Read the model definition and answer for the solid it produces. Units are mm, in the model's axes. Coordinates: 2 decimals unless noted, no trailing zeros. Write each loop counter-clockwise with the first axis right and the second up, starting at its lowest first coordinate (ties: lowest second). Pieces come first, ordered by that corner, then holes.
(1) Given pin 1 (1 mm diameter, centred on x = -2.5, y = 0.5, fed in from +Z); pin 2 (1 mm diameter, centred on x = -8, y = 2.5, fed in from -Z), each flat-ended and moving along its own axis, determine where each tip first touches the part or whether it passes through.
(2) Find the intervals of material crossed by probe 1 along Z at (x, y) = (-21.5, 1.8); probe 2 along Z at (x, y) = (-3, 1.55); probe 3 along X at (y, z) = (0.6, -132.5), in increasing order.
(3) Section B-B on x = -26.5 is taken. Write down the section's boundary in (y, z).
Autodesk Inventor part; units mm, degrees
ref_plane "YZ Plane" through (0, 0, 0) normal (1, 0, 0) x (0, 1, 0)
ref_plane "XZ Plane" through (0, 0, 0) normal (0, 1, 0) x (-1, 0, 0)
ref_plane "XY Plane" through (0, 0, 0) normal (0, 0, 1) x (1, 0, 0)
sketch "Sketch1" plane through (0, 0, 0) normal (0, 1, 0) x (-1, 0, 0)
  line L0 (0, 0) -> (-30, 0)
  line L1 (-30, 0) -> (-30, -140)
  line L2 (-30, -140) -> (0, -140)
  line L3 (0, -140) -> (0, 0)
  line L4 (0, 0) -> (0, -10)
  line L5 (0, -10) -> (40, -10)
  line L6 (40, -10) -> (40, -130)
  line L7 (40, -130) -> (0, -130)
  line L8 (0, -130) -> (0, -10)
  point P0 (0, -130)
  dimension "d0" = 30
  dimension "d1" = 140
  dimension "d2" = 10
  dimension "d3" = 40
  dimension "d4" = 120
extrude "Extrusion1" add sketch "Sketch1" along normal blind 3
fillet "Fillet1" radius 10 2 edges at (0, 1.5, -10) (0, 1.5, -130)
properties part number "lateral_base"
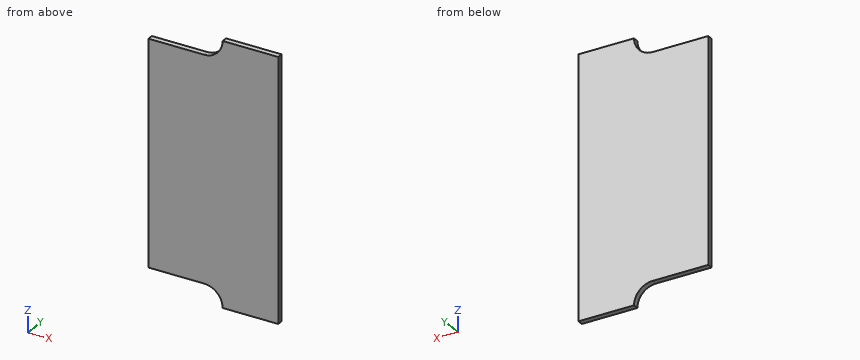
Response:
1. pin 1: stops at z = -6
1. pin 2: stops at z = -130.32
2. probe 1: z = -130 to -10
2. probe 2: z = -132.86 to -7.14
2. probe 3: x = -3.39 to 30
3. outline: (0, -130) - (3, -130) - (3, -10) - (0, -10) - close
